Source: three-view drawing plus pictorial views. Frame: mm from the lowest corner of the part. Give positions to 0.01 mm unless a question says otherwise; leave off trailing zeros. Loops run counter-clockwise (first coordinate to the right, second up) from the corner with the lowest first, then second, coordinate; pieces in that order, holes last. Notation, with made-up numbers: (37.5, -12.75) - (86.5, -12.75) arc R24 cw to (86.5, -0.75) - close; hole circle Ø8 at (15.5, 71). An arc over 180 degrees is marked (long way). Answer as a JSON object with one key per item and string values.
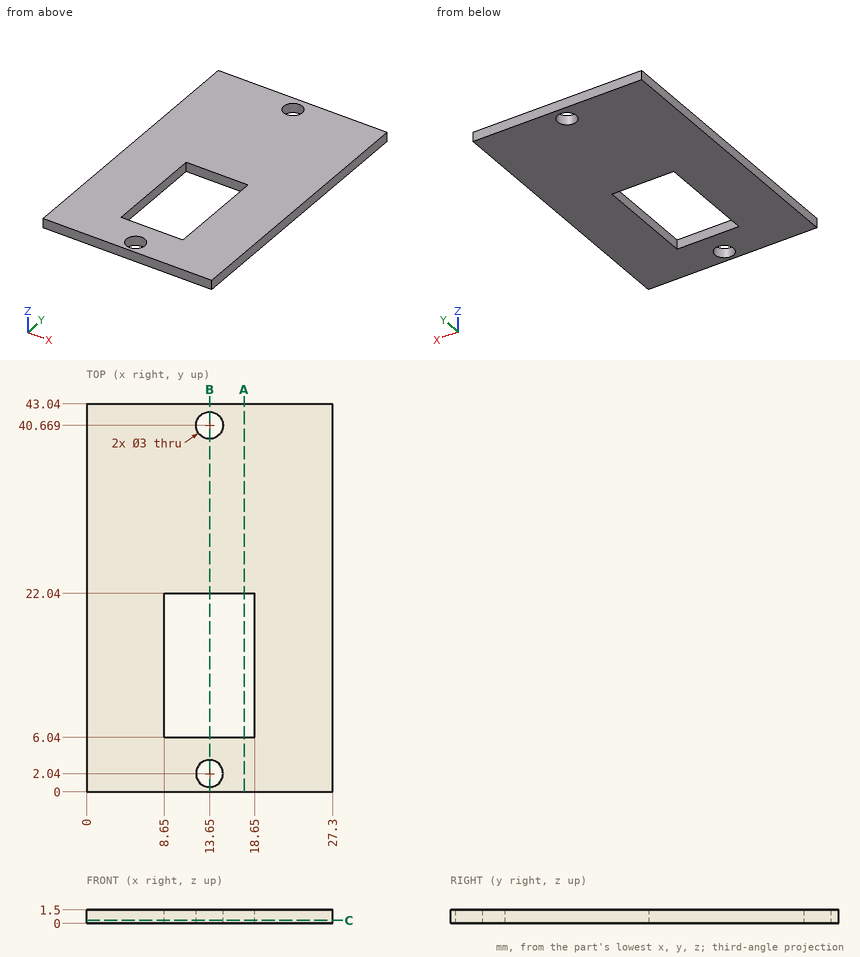
Item 1: Cut plane B-B (x = 13.65). Return loops of the section in (y, z).
Geometry check:
{"outline": "(0, 0) - (0.54, 0) - (0.54, 1.5) - (0, 1.5) - close; (3.54, 0) - (6.04, 0) - (6.04, 1.5) - (3.54, 1.5) - close; (22.04, 0) - (39.17, 0) - (39.17, 1.5) - (22.04, 1.5) - close; (42.17, 0) - (43.04, 0) - (43.04, 1.5) - (42.17, 1.5) - close"}
Item 2: Material intervals for line 1 (Y direction, x = 13.65, z = 0.8); line 2 (X direction, y = 2, z = 0.6); line 3 (X direction, y = 15.5, z = 0.3), sorted ascending. Write a range as [from, to].
Geometry check:
{"line 1": "y = [0, 0.54], [3.54, 6.04], [22.04, 39.17], [42.17, 43.04]", "line 2": "x = [0, 12.15], [15.15, 27.3]", "line 3": "x = [0, 8.65], [18.65, 27.3]"}
Item 3: Cut plane A-A (x = 17.5). Return loops of the section in (y, z).
Geometry check:
{"outline": "(0, 0) - (6.04, 0) - (6.04, 1.5) - (0, 1.5) - close; (22.04, 0) - (43.04, 0) - (43.04, 1.5) - (22.04, 1.5) - close"}
Item 4: Cut plane C-C (z = 0.35). Return loops of the section in (x, y), then the cut area to 3 significant figures.
Geometry check:
{"outline": "(0, 0) - (27.3, 0) - (27.3, 43.04) - (0, 43.04) - close; hole (8.65, 6.04) - (18.65, 6.04) - (18.65, 22.04) - (8.65, 22.04) - close; hole circle Ø3 at (13.65, 2.04); hole circle Ø3 at (13.65, 40.67)", "area": "1,000 mm2"}
